Here's how the part is built. I have some questions about the finished solid (model axes, mm). A direction names the side the tool comes from. Round coordinates to 2 decimals unless told otherwise and drop trailing zeros. Loops run counter-clockwise (first coordinate to the right, second up) from the corner with the lowest first, then second, coordinate; pieces in that order, holes last. Notation, with made-up numbers: M -4.5,63 L 53.5,63 A16 cw 53.5,70 Z; hole C 41.5,10.25 d1. An arc over 180 degrees is marked long. Use a Markdown table: item, result.
```python
from build123d import *

# Parameters (mm, degrees)
BOSS_EXTRUDE2_DEPTH = 25.4
BOSS_EXTRUDE2_DRAFT = -0.5
CUT_EXTRUDE1_DEPTH  = 24.13
CUT_EXTRUDE1_DRAFT  = -0.5
FILLET1_R           = 6.35
FILLET2_R           = 6.35
SKETCH7_R           = 21.209
BOSS_EXTRUDE3_DEPTH = 25.4
BOSS_EXTRUDE3_TAPER = 5
SKETCH11_R          = 18.415
CUT_EXTRUDE2_DEPTH  = 26.67
CUT_EXTRUDE2_DRAFT  = 0.5
FILLET3_R           = 5.08
FILLET4_R           = 5.08


with BuildPart() as part:
    # Sketch5 → Boss-Extrude2 (with draft: the straight prism first)
    with BuildSketch(Plane(origin=(0, 0, 0), x_dir=(1, 0, 0), z_dir=(0, 1, 0))):
        with BuildLine():
            ThreePointArc((-26.568599378, 32.36603099), (-40.038983559, 26.786415172), (-45.618599378, 13.31603099))
            Line((-45.618599378, 13.31603099), (-45.618599378, -24.78396901))
            ThreePointArc((-45.618599378, -24.78396901), (-40.038983559, -38.254353191), (-26.568599378, -43.83396901))
            Line((-26.568599378, -43.83396901), (36.931400622, -43.83396901))
            ThreePointArc((36.931400622, -43.83396901), (50.401784804, -38.254353191), (55.981400622, -24.78396901))
            Line((55.981400622, -24.78396901), (55.981400622, 13.31603099))
            ThreePointArc((55.981400622, 13.31603099), (50.401784804, 26.786415172), (36.931400622, 32.36603099))
            Line((36.931400622, 32.36603099), (-26.568599378, 32.36603099))
        make_face()
    extrude(amount=-BOSS_EXTRUDE2_DEPTH)
    # Boss-Extrude2: the draft: its side faces are tilted about the plane it starts from
    boss_extrude2_sides = [part.faces().sort_by_distance(p)[0] for p in [
        (-40.038983559, -12.7, -26.786415172),
        (-45.618599378, -12.7, 5.73396901),
        (-40.038983559, -12.7, 38.254353191),
        (5.181400622, -12.7, 43.83396901),
        (50.401784804, -12.7, 38.254353191),
        (55.981400622, -12.7, 5.73396901),
        (50.401784804, -12.7, -26.786415172),
        (5.181400622, -12.7, -32.36603099),
    ]]
    draft(boss_extrude2_sides, Plane(origin=(0, 0, 0), x_dir=(1, 0, 0), z_dir=(0, 1, 0)), BOSS_EXTRUDE2_DRAFT)


with BuildPart() as cut_extrude1_tool:
    # Sketch6 → Cut-Extrude1 (with draft: the straight prism first)
    with BuildSketch(Plane(origin=(0, 0, 0), x_dir=(1, 0, 0), z_dir=(0, 1, 0))):
        with BuildLine():
            ThreePointArc((-25.933599378, 31.73103099), (-39.403983559, 26.151415172), (-44.983599378, 12.68103099))
            Line((-44.983599378, 12.68103099), (-44.983599378, -24.14896901))
            ThreePointArc((-44.983599378, -24.14896901), (-39.403983559, -37.619353191), (-25.933599378, -43.19896901))
            Line((-25.933599378, -43.19896901), (36.296400622, -43.19896901))
            ThreePointArc((36.296400622, -43.19896901), (49.766784804, -37.619353191), (55.346400622, -24.14896901))
            Line((55.346400622, -24.14896901), (55.346400622, 12.68103099))
            ThreePointArc((55.346400622, 12.68103099), (49.766784804, 26.151415172), (36.296400622, 31.73103099))
            Line((36.296400622, 31.73103099), (-25.933599378, 31.73103099))
        make_face()
    extrude(amount=-CUT_EXTRUDE1_DEPTH)
    # Cut-Extrude1: the draft: its side faces are tilted about the plane it starts from
    cut_extrude1_sides = [cut_extrude1_tool.faces().sort_by_distance(p)[0] for p in [
        (-39.403983559, -12.065, -26.151415172),
        (-44.983599378, -12.065, 5.73396901),
        (-39.403983559, -12.065, 37.619353191),
        (5.181400622, -12.065, 43.19896901),
        (49.766784804, -12.065, 37.619353191),
        (55.346400622, -12.065, 5.73396901),
        (49.766784804, -12.065, -26.151415172),
        (5.181400622, -12.065, -31.73103099),
    ]]
    draft(cut_extrude1_sides, Plane(origin=(0, 0, 0), x_dir=(1, 0, 0), z_dir=(0, 1, 0)), CUT_EXTRUDE1_DRAFT)


with BuildPart() as part_1:
    add(part.part)

    # Cut-Extrude1: cut by cut_extrude1_tool
    add(cut_extrude1_tool.part, mode=Mode.SUBTRACT)

    # Fillet1
    fillet1_edges = [part_1.edges().sort_by_distance(p)[0] for p in [
        (-39.882244543, -25.4, -26.629676156),
        (-45.396936936, -25.4, 5.73396901),
        (-39.882244543, -25.4, 38.097614176),
        (5.181400622, -25.4, 43.612306568),
        (50.245045788, -25.4, 38.097614176),
        (55.759738181, -25.4, 5.73396901),
        (50.245045788, -25.4, -26.629676156),
        (5.181400622, -25.4, -32.144368548),
    ]]
    fillet(fillet1_edges, radius=FILLET1_R)

    # Fillet2
    fillet2_edges = [part_1.edges().sort_by_distance(p)[0] for p in [
        (-39.255081494, -24.13, 37.470451126),
        (-44.773020058, -24.13, 5.73396901),
        (-39.255081494, -24.13, -26.002513107),
        (5.181400622, -24.13, -31.52045167),
        (49.617882739, -24.13, -26.002513107),
        (55.135821303, -24.13, 5.73396901),
        (49.617882739, -24.13, 37.470451126),
        (5.181400622, -24.13, 42.98838969),
    ]]
    fillet(fillet2_edges, radius=FILLET2_R)

    # Sketch7 → Boss-Extrude3 (add)
    with BuildSketch(Plane.XZ.offset(25.4)):
        with Locations((5.181400622, 5.73396901)):
            Circle(SKETCH7_R)
    extrude(amount=BOSS_EXTRUDE3_DEPTH, taper=BOSS_EXTRUDE3_TAPER)


with BuildPart() as cut_extrude2_tool:
    # Sketch11 → Cut-Extrude2 (with draft: the straight prism first)
    with BuildSketch(Plane.XZ.offset(50.8)):
        with Locations((5.181400622, 5.73396901)):
            Circle(SKETCH11_R)
    extrude(amount=-CUT_EXTRUDE2_DEPTH)
    # Cut-Extrude2: the draft: its side faces are tilted about the plane it starts from
    cut_extrude2_sides = [cut_extrude2_tool.faces().sort_by_distance(p)[0] for p in [
        (-13.233599378, -37.465, 5.73396901),
    ]]
    draft(cut_extrude2_sides, Plane.XZ.offset(50.8), CUT_EXTRUDE2_DRAFT)


with BuildPart() as part_2:
    add(part_1.part)

    # Cut-Extrude2: cut by cut_extrude2_tool
    add(cut_extrude2_tool.part, mode=Mode.SUBTRACT)

    # Fillet3
    fillet3_edges = [part_2.edges().sort_by_distance(p)[0] for p in [
        (-13.466344942, -24.13, 5.73396901),
    ]]
    fillet(fillet3_edges, radius=FILLET3_R)

    # Fillet4
    fillet4_edges = [part_2.edges().sort_by_distance(p)[0] for p in [
        (-16.027599378, -25.4, 5.73396901),
    ]]
    fillet(fillet4_edges, radius=FILLET4_R)


solid = part_2.part
```
Q1. For faces 1 (the conical face through (-40.128, -9.419, 38.048)), 2 (the flat face through (5, -25.4, 33)), 3 (the conical face through (-39.833, -9.419, -26.875)), 4 (the cylindrical face through (4.746, -22.241, -29.745)), which set-ups out of +Z, -Z, +X, -X, +Y, -Y let a thin tool reach every point of the face, with its end or its side?
Return value:
| item | result |
|---|---|
| face 1 | +Z, -X, -Y |
| face 2 | -Y |
| face 3 | -Z, -X, -Y |
| face 4 | +Y |
Q2. Imagine slicing it at A-A, the plane y = -9. Please give me the cut outline in (x, z), then the cut area to 3 significant figures.
Return value:
| item | result |
|---|---|
| outline | M -45.54,-13.32 A18.97 ccw -26.57,-32.29 L 36.93,-32.29 A18.97 ccw 55.9,-13.32 L 55.9,24.78 A18.97 ccw 36.93,43.76 L -26.57,43.76 A18.97 ccw -45.54,24.78 Z; hole M -44.91,-12.68 A18.97 ccw -25.93,-31.65 L 36.3,-31.65 A18.97 ccw 55.27,-12.68 L 55.27,24.15 A18.97 ccw 36.3,43.12 L -25.93,43.12 A18.97 ccw -44.91,24.15 Z |
| area | 224 mm^2 |
Q3. Imagine slicing it at B-B, the plane y = -21.5. Please give me the cut outline in (x, z), then the cut area to 3 significant figures.
Return value:
| item | result |
|---|---|
| outline | M -44.96,-13.32 A18.39 ccw -26.57,-31.71 L 36.93,-31.71 A18.39 ccw 55.32,-13.32 L 55.32,24.78 A18.39 ccw 36.93,43.18 L -26.57,43.18 A18.39 ccw -44.96,24.78 Z; hole M -43.62,-12.68 A17.69 ccw -25.93,-30.37 L 36.3,-30.37 A17.69 ccw 53.99,-12.68 L 53.99,24.15 A17.69 ccw 36.3,41.84 L -25.93,41.84 A17.69 ccw -43.62,24.15 Z |
| area | 439 mm^2 |
Q4. I need wall thicknesses on line 1 (Z direction, x = 14, y = -18); line 2 (X direction, y = -17.5, z = 16); line 3 (X direction, y = -3, z = -10). Which ranges of each line are inside material? Lowest first, please. Write a range as from..to.
Return value:
| item | result |
|---|---|
| line 1 | z = -32.21..-31.57, 43.04..43.68 |
| line 2 | x = -45.47..-44.83, 55.19..55.83 |
| line 3 | x = -45.59..-44.96, 55.32..55.96 |
Q5. Will these pins go through, and if not, where does the flat tip stop? P1, Ø10, axis at x = 36.5, z = -20, coming from the -Y side; P2, Ø10, axis at x = 6.5, z = -7.5, coming from the -Y side; P3, Ø5, axis at x = 13.5, y = -17, coming from the -Z side; P4, Ø2, axis at x = -20.5, y = -13, coming from the -Z side.
Return value:
| item | result |
|---|---|
| P1 | stops at y = -25.4 |
| P2 | passes through |
| P3 | stops at z = -32.24 |
| P4 | stops at z = -32.26 |
Q6. We'd pull the mould along X, two halves only. Please class faces 5 (the flat face through (-13.2, -50.8, 8.6)), 6 (the cylindrical face through (-43, -22.24, 5.99)), 7 (the cylindrical face through (53.984, -23.511, 5.467)), 8 (the conical face through (49.86, -8.79, -25.95)): pulls with the +X half, pulls with the -X half, needs draft (parallel to the pull), parting line crosses it, or undercut.
Return value:
| item | result |
|---|---|
| face 5 | needs draft |
| face 6 | undercut |
| face 7 | pulls with the +X half |
| face 8 | undercut |
Q7. Imagine slicing it at C-C, the plane y = -45. Please give me the cut outline in (x, z).
Return value:
| item | result |
|---|---|
| outline | C 5.18,5.73 d38.99; hole C 5.18,5.73 d36.93 |
